Verification items for this drawing (mm, ordinates from the low corner). A direction names the side the tool comes from. Coordinates: 2 decimals unless noted, no trailing zeros. Loops run counter-clockwise (first coordinate to the right, second up) from the corner with the lowest first, then second, coordinate; pieces in that order, holes last. Notation, with made-up numbers: (48, 64) - (59, 64) arc R15 ccw to (59, 78) - close; hole circle Ø10 at (14, 56). An arc over 180 degrees is marked (long way). Write each question's results on one line, items separated by ' | '. Start each with the question number.
(1) Sectioned sample at B-B (x = 40). Enter the section's corners in (y, z).
(2) Access from +Z, -Z, +X, -X, +Y, -Y to the whole of each face (thin tool, end or side, straight path). Record for the marked faces 1, 2 and 3.
(3) Go/stop test with flat-tipped pins: pin 1 Ø5 at (y, z) = (26, 33.5) entering from +X; pin 2 Ø3 at (x, z) = (27, 23) entering from +Y; pin 3 Ø5 at (x, y) = (23, 30.5) entering from -Z. Record where each tip stops, or that it passes through.
(4) Material ranges on probe 1 along X at (y, z) = (23, 35); probe 2 along Y at (x, z) = (12, 16.5); probe 3 along Z at (x, y) = (37.5, 24) (1 decimal), recorded low to high.
(5) Sectioned sample at A-A (x = 23). Enter the section's corners in (y, z), plus the area to 3 significant figures.
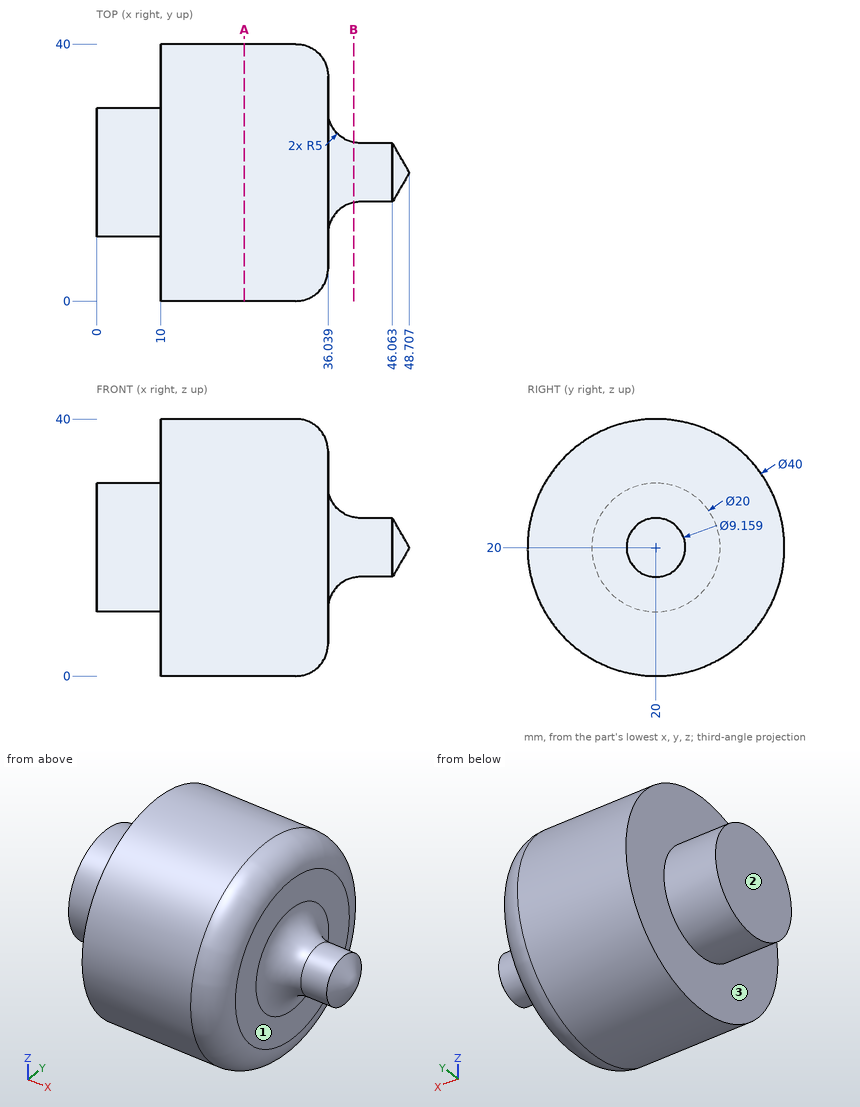
Outcome:
1) outline: circle Ø9.38 at (20, 20)
2) face 1: +X | face 2: +Z, -Z, -X, +Y, -Y | face 3: -X
3) pin 1: stops at x = 36.04 | pin 2: stops at y = 39.94 | pin 3: stops at z = 1.67
4) probe 1: x = 10 to 36.03 | probe 2: y = 0.31 to 39.69 | probe 3: z = 15.5 to 24.5
5) outline: circle Ø40 at (20, 20) | area: 1,260 mm2
